Input: part model. Units: mm. Frame: model coordinates. Coordinates: 2 decimals unless noted, no trailing zeros. Order: outer loops, then holes, each group sorted by start corner. A loop starts at its lowest first (then second) coordinate and runs counter-clockwise, first axis right, second up. Notation, with made-up numbers: (40.25, 52.5) -> (90.25, 52.5) arc R32 cw to (90.25, 83.5) -> close; hole circle Ø8 at (-21, 33). An arc over 180 degrees is marked (long way). Answer as CSV lines item,"result".
from build123d import *

# Parameters (mm, degrees)
SKETCH2_R                    = 1.5
SKETCH2_R_2                  = 2.5
BOSS_EXTRUDE1_DEPTH          = 12.2
CUT_EXTRUDE_THIN2_DEPTH      = 82.319370386
CUT_EXTRUDE_THIN2_DEPTH_BACK = 60
CUT_EXTRUDE_THIN3_DEPTH      = 82.314797438
CUT_EXTRUDE_THIN3_DEPTH_BACK = 10
SKETCH4_W                    = 1
SKETCH4_H                    = 38.438218158


with BuildPart() as part:
    # Sketch2 → Boss-Extrude1 (new body)
    with BuildSketch(Plane.XY):
        with BuildLine():
            Line((-8, -72), (-6, 74))
            ThreePointArc((-6, 74), (0, 80), (6, 74))
            Line((6, 74), (8, -72))
            ThreePointArc((8, -72), (0, -80), (-8, -72))
        make_face()
        with Locations((0, 74)):
            Circle(SKETCH2_R, mode=Mode.SUBTRACT)
        with Locations((0, -62)):
            Circle(SKETCH2_R_2, mode=Mode.SUBTRACT)
    extrude(amount=BOSS_EXTRUDE1_DEPTH)

    # Sketch3 → Cut-Extrude-Thin2 (cut, two sides: drawn at the far end of the back side and taken through both)
    with BuildSketch(Plane.XY.offset(12.2).offset(-CUT_EXTRUDE_THIN2_DEPTH_BACK)):
        with BuildLine():
            ThreePointArc((-7.952635689, -68.542405266), (0, -76.6047273), (7.952635689, -68.542405266))
            Line((7.952635689, -68.542405266), (17.951697558, -68.405431815))
            ThreePointArc((17.951697558, -68.405431815), (0, -86.6047273), (-17.951697558, -68.405431815))
            Line((-17.951697558, -68.405431815), (-7.952635689, -68.542405266))
        make_face()
    extrude(amount=CUT_EXTRUDE_THIN2_DEPTH + CUT_EXTRUDE_THIN2_DEPTH_BACK, mode=Mode.SUBTRACT)

    # Sketch4 → Cut-Extrude-Thin3 (cut, two sides: drawn at the far end of the back side and taken through both)
    with BuildSketch(Plane.XY.offset(12.2).offset(-CUT_EXTRUDE_THIN3_DEPTH_BACK)):
        with Locations((0, 34.719285659)):
            Rectangle(SKETCH4_W, SKETCH4_H)
    extrude(amount=CUT_EXTRUDE_THIN3_DEPTH + CUT_EXTRUDE_THIN3_DEPTH_BACK, mode=Mode.SUBTRACT)


solid = part.part
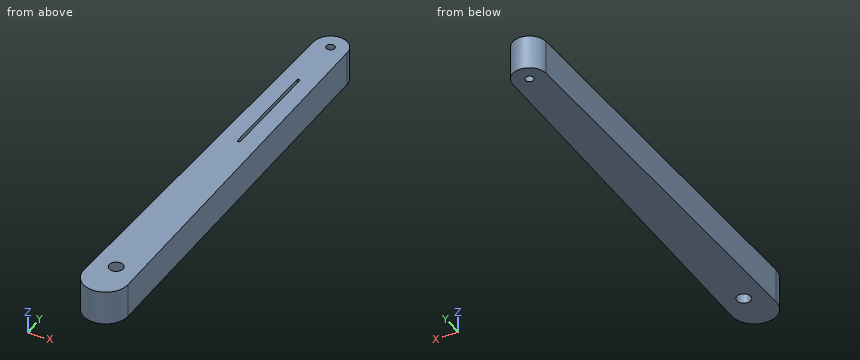
1. Ray query, line 1 along Y through (x, z) = (0, 4.5); line 2 along X through (y, z) = (74, 9.5); line 3 along Y through (x, z) = (-1.75, 5.25). Return the intervals inside material, ascending.
Findings:
line 1,"y = -76.6 to -64.5, -59.5 to 15.5, 53.94 to 72.5, 75.5 to 80"
line 2,"x = -6 to -1.5, 1.5 to 6"
line 3,"y = -76.41 to -63.79, -60.21 to 79.74"
2. Cut plane C-C (y = 39). Return the cut outline in (x, z), plus the area to 3 significant figures.
Findings:
outline,"(-6.48, 0) -> (6.48, 0) -> (6.48, 12.2) -> (0.5, 12.2) -> (0.5, 2.2) -> (-0.5, 2.2) -> (-0.5, 12.2) -> (-6.48, 12.2) -> close"
area,"148 mm2"
3. Cut plane A-A (z = 7.25). Return the cut outline in (x, y), plus the area to 3 significant figures.
Findings:
outline,"(-7.95, -68.54) arc R7.95 ccw (long way) to (7.95, -68.54) -> (6, 74) arc R6 ccw to (-6, 74) -> close; hole circle Ø5 at (0, -62); hole circle Ø3 at (0, 74); hole (-0.5, 15.5) -> (0.5, 15.5) -> (0.5, 53.94) -> (-0.5, 53.94) -> close"
area,"2,080 mm2"
4. Contact query for flat-ended pins moving along their axis: pin 1 (0.5 mm diameter, centred on x = 0, y = 39, fed in from +Z); pin 2 (5 mm diameter, centred on x = 0, y = 74, fed in from +Z); pin 3 (5 mm diameter, centred on x = -5, z = 4, fed in from +Y); pin 4 (3 mm diameter, centred on y = 28.5, z = 9.5, fed in from -X). Output: stop coordinate, or through.
Findings:
pin 1,"stops at z = 2.2"
pin 2,"stops at z = 12.2"
pin 3,"stops at y = 79.45"
pin 4,"stops at x = -6.64"
5. Cut plane D-D (x = 4.25). Return the cut outline in (y, z), plus the area to 3 significant figures.
Findings:
outline,"(-75.37, 0) -> (78.24, 0) -> (78.24, 12.2) -> (-75.37, 12.2) -> close"
area,"1,870 mm2"
6. Cut plane B-B (y = -62). Return the cut outline in (x, z).
Findings:
outline,"(-7.86, 0) -> (-2.5, 0) -> (-2.5, 12.2) -> (-7.86, 12.2) -> close; (2.5, 0) -> (7.86, 0) -> (7.86, 12.2) -> (2.5, 12.2) -> close"
